Design review of the part shown in the three views and the two pictorial views. Dimensions are in mm from the part's minimum x, y and z. Give positions to 0.01 mm unless a question says otherwise; leave off trailing zeros. Loops run counter-clockwise (first coordinate to the right, second up) from the corner with the lowest first, then second, coordinate; pieces in that order, holes last. Notation, with made-up numbers: (61, 87) - (90, 87) arc R19 ccw to (90, 95) - close; hole circle Ø5 at (80, 47). An arc over 180 degrees is marked (long way). Return JSON: item names as keys, results as strings. Group by question number.
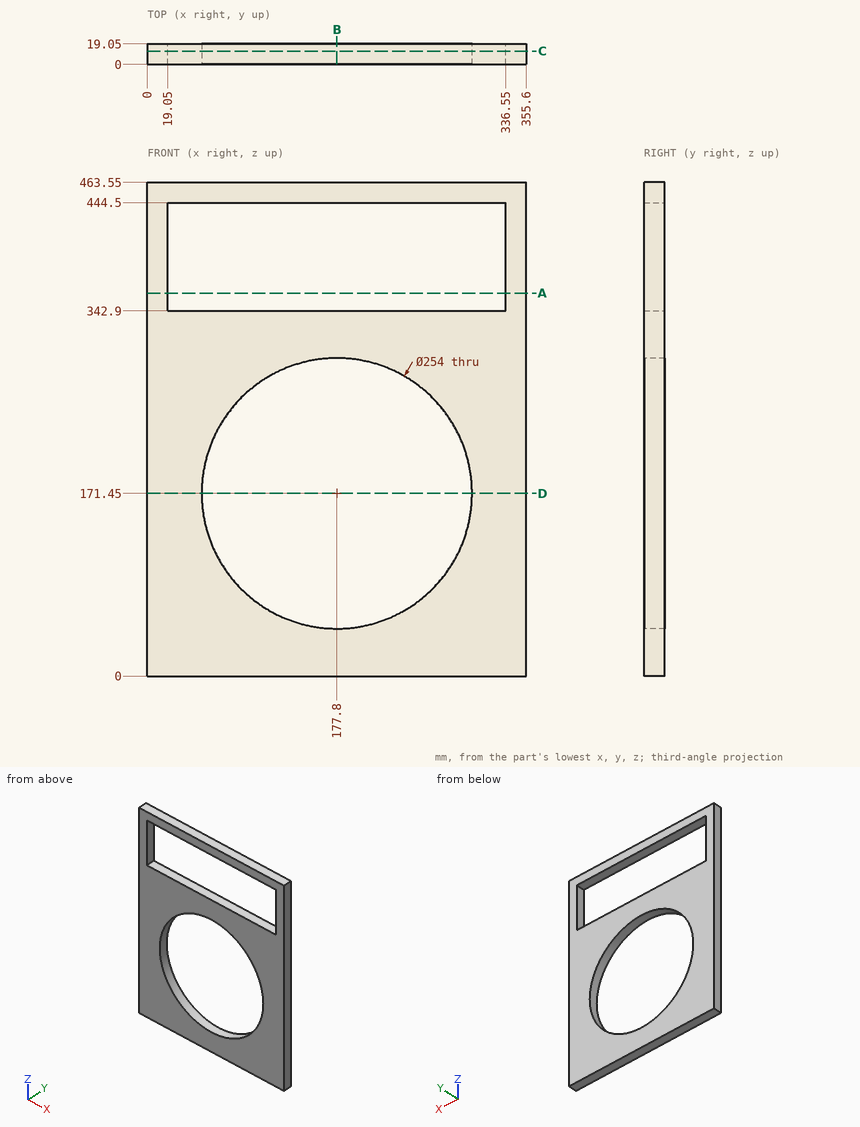
Item 1: Take a section at B-B (x = 177.8). State the section outline as (y, z) points.
Item 2: Take a section at D-D (z = 171.45). State the section outline as (x, y) points.
Item 3: Take a section at A-A (z = 359.5). State the section outline as (x, y) points, then the cut area to 3 significant figures.
Item 4: Take a section at C-C (y = 12.25). State the section outline as (x, z) points, then the cut area to 3 significant figures.
Item 5: For L1, parallel to Z at x = 177.8, y = 9.25; L2, parallel to X at y = 8, z = 434.5; L3, parallel to Z at x = 229.5, y = 1.5, list the stretches that pass through material, from the lowest coordinate up. Write a range as from..to.
Item 6: For P1, Ø9.5, axis at x = 128, y = 7, coming from the -Z side, flat-tipped, find the tip position at first contact; note if it passes through.
Check sheet entries:
{
 "1": {"outline": "(0, 0) - (19.05, 0) - (19.05, 44.45) - (0, 44.45) - close; (0, 298.45) - (19.05, 298.45) - (19.05, 342.9) - (0, 342.9) - close; (0, 444.5) - (19.05, 444.5) - (19.05, 463.55) - (0, 463.55) - close"},
 "2": {"outline": "(0, 0) - (50.8, 0) - (50.8, 19.05) - (0, 19.05) - close; (304.8, 0) - (355.6, 0) - (355.6, 19.05) - (304.8, 19.05) - close"},
 "3": {"outline": "(0, 0) - (19.05, 0) - (19.05, 19.05) - (0, 19.05) - close; (336.55, 0) - (355.6, 0) - (355.6, 19.05) - (336.55, 19.05) - close", "area": "726 mm^2"},
 "4": {"outline": "(0, 0) - (355.6, 0) - (355.6, 463.55) - (0, 463.55) - close; hole (19.05, 342.9) - (336.55, 342.9) - (336.55, 444.5) - (19.05, 444.5) - close; hole circle Ø254 at (177.8, 171.45)", "area": "81,900 mm^2"},
 "5": {"L1": "z = 0..44.45, 298.45..342.9, 444.5..463.55", "L2": "x = 0..19.05, 336.55..355.6", "L3": "z = 0..55.45, 287.45..342.9, 444.5..463.55"},
 "6": {"P1": "stops at z = 0"}
}
